```python
from build123d import *

# Parameters (mm, degrees)
ESQUISSE1_W             = 20
ESQUISSE1_H             = 7
ESQUISSE1_W_2           = 7
ESQUISSE1_H_2           = 51.9
BOSS_EXTRU_1_DEPTH      = 9
ESQUISSE2_R             = 1.8
ENL_V_MAT_EXTRU_1_DEPTH = 9
ESQUISSE3_R             = 1.8
ENL_V_MAT_EXTRU_2_DEPTH = 9


with BuildPart() as part:
    # Esquisse1 → Boss.-Extru.1 (new body)
    with BuildSketch(Plane.XY):
        with Locations((10, 3.5)):
            Rectangle(ESQUISSE1_W, ESQUISSE1_H)
        with Locations((16.5, 32.95)):
            Rectangle(ESQUISSE1_W_2, ESQUISSE1_H_2)
    extrude(amount=BOSS_EXTRU_1_DEPTH)

    # Esquisse2 → Enlèv. mat.-Extru.1 (cut)
    with BuildSketch(Plane(origin=(0, 7, 0), x_dir=(1, 0, 0), z_dir=(0, 1, 0))):
        with Locations(Location((10, -4.5, 0), (0, 0, 270))):
            Circle(ESQUISSE2_R)
    extrude(amount=-ENL_V_MAT_EXTRU_1_DEPTH, mode=Mode.SUBTRACT)

    # Esquisse3 → Enlèv. mat.-Extru.2 (cut)
    with BuildSketch(Plane.ZY.offset(-13)):
        with Locations(Location((4.5, 53.9, 0), (0, 0, 270))):
            Circle(ESQUISSE3_R)
    extrude(amount=-ENL_V_MAT_EXTRU_2_DEPTH, mode=Mode.SUBTRACT)


solid = part.part
```
CAD build for the part. Positions are in the model's coordinates, mm. A direction names the side the tool comes from. Round coordinates to 2 decimals unless told otherwise and drop trailing zeros. Loops run counter-clockwise (first coordinate to the right, second up) from the corner with the lowest first, then second, coordinate; pieces in that order, holes last. Notation, with made-up numbers: M -19,60 L -11,60 A9 cw -11,68 Z; hole C 1.5,-1 d10. An arc over 180 degrees is marked long. Return JSON: item names as keys, results as strings. Group by question number.
(1) Drop flat-ended pins along their axis: P1, Ø1, axis at y = 10, z = 1.5, coming from the -X side; P2, Ø1, axis at x = 9.5, z = 3.5, coming from the -Y side. Give the stop position or say it passes through.
(2) Saw through at B-B, the plane x = 10. List the corners of the cut face in (y, z).
(3) Saw through at A-A, the plane y = 53.9. List the corners of the cut face in (x, z).
(4) Saw through at C-C, the plane x = 16. List the corners of the cut face in (y, z), and give its area (3 significant figures).
(5) Saw through at D-D, the plane z = 5.5. List the corners of the cut face in (x, y), and give its area (3 significant figures).
(6) Wall check: probe 1 along X at (y, z) = (2, 4.5); probe 2 along Z at (x, y) = (16.5, 53.9); probe 3 along X at (y, z) = (32, 6.75). Give the ranges that are in metal, low to high. Write a range as [from, to].
(7) Tool access for faces 1 (the flat face through (13, 33, 4)), 2 (the flat face through (16, 58.9, 4)): list every direction of +Z, -Z, +X, -X, +Y, -Y with a clear straight run to the whole face (end or side of a thin tool).
(8) Mould opens along Z. For faces 3 (the flat face through (14, 23, 0)), 4 (the cylindrical face through (8.243, 3.549, 4.11)), 5 (the flat face through (6, 7, 4)) say: +Z half, -Z half, draft (parallel to the pull), parting line (faces both ways), or undercut.
Answer list:
{
 "1": {"P1": "x = 13", "P2": "through"},
 "2": {"outline": "M 0,0 L 7,0 L 7,2.7 L 0,2.7 Z; M 0,6.3 L 7,6.3 L 7,9 L 0,9 Z"},
 "3": {"outline": "M 13,0 L 20,0 L 20,2.7 L 13,2.7 Z; M 13,6.3 L 20,6.3 L 20,9 L 13,9 Z"},
 "4": {"outline": "M 0,0 L 58.9,0 L 58.9,9 L 0,9 Z; hole C 53.9,4.5 d3.6", "area": "520 mm2"},
 "5": {"outline": "M 0,0 L 8.5,0 L 8.5,7 L 0,7 Z; M 11.5,0 L 20,0 L 20,52.4 L 13,52.4 L 13,7 L 11.5,7 Z; M 13,55.4 L 20,55.4 L 20,58.9 L 13,58.9 Z", "area": "461 mm2"},
 "6": {"probe 1": "[0, 8.2], [11.8, 20]", "probe 2": "[0, 2.7], [6.3, 9]", "probe 3": "[13, 20]"},
 "7": {"face 1": "+Z, -Z, -X, +Y", "face 2": "+Z, -Z, +X, -X, +Y"},
 "8": {"face 3": "-Z half", "face 4": "undercut", "face 5": "draft"}
}
